from build123d import *

# Parameters (mm, degrees)
BOSS_EXTRUDE1_DEPTH = 4
SKETCH4_R           = 1.5
CUT_EXTRUDE1_DEPTH  = 3
SKETCH5_R           = 1.5
CUT_EXTRUDE2_DEPTH  = 3
SKETCH6_W           = 14.4
SKETCH6_H           = 0.4
CUT_EXTRUDE3_DEPTH  = 4
FILLET1_R           = 1
FILLET2_R           = 2


with BuildPart() as part:
    # Sketch3 → Boss-Extrude1 (new body)
    with BuildSketch(Plane(origin=(0, 0, 0), x_dir=(0, 1, 0), z_dir=(0, 0, 1))):
        with BuildLine():
            Line((-34.7, -0.521026003), (-34.7, -2.457826354))
            ThreePointArc((-34.7, -2.457826354), (-37.7, -4.907316097), (-34.7, -7.35680584))
            Line((-34.7, -7.35680584), (-34.7, -9.880280288))
            Line((-34.7, -9.880280288), (-34.7, -32.518065271))
            ThreePointArc((-34.7, -32.518065271), (-37.5, -35), (-34.7, -37.481934729))
            Line((-34.7, -37.481934729), (-34.7, -42.857826354))
            ThreePointArc((-34.7, -42.857826354), (-37.7, -45.307316097), (-34.7, -47.75680584))
            Line((-34.7, -47.75680584), (-34.7, -48.807316097))
            Line((-34.7, -48.807316097), (34.7, -48.807316097))
            Line((34.7, -48.807316097), (34.7, -47.75680584))
            ThreePointArc((34.7, -47.75680584), (37.7, -45.307316097), (34.7, -42.857826354))
            Line((34.7, -42.857826354), (34.7, -37.481934729))
            ThreePointArc((34.7, -37.481934729), (37.5, -35), (34.7, -32.518065271))
            Line((34.7, -32.518065271), (34.7, -7.35680584))
            ThreePointArc((34.7, -7.35680584), (37.7, -4.907316097), (34.7, -2.457826354))
            Line((34.7, -2.457826354), (34.7, -0.521026003))
            Line((34.7, -0.521026003), (6.445103659, -0.521026003))
            ThreePointArc((6.445103659, -0.521026003), (4, 2.5), (1.554896341, -0.521026003))
            Line((1.554896341, -0.521026003), (-1.554896341, -0.521026003))
            ThreePointArc((-1.554896341, -0.521026003), (-4, 2.5), (-6.445103659, -0.521026003))
            Line((-6.445103659, -0.521026003), (-34.7, -0.521026003))
        make_face()
        Polygon((-32.7, -9.880280288), (-32.7, -46.807316097), (32.7, -46.807316097), (32.7, -2.521026003), (-32.7, -2.521026003), align=None, mode=Mode.SUBTRACT)
    extrude(amount=BOSS_EXTRUDE1_DEPTH)

    # Sketch4 → Cut-Extrude1 (cut)
    with BuildSketch(Plane.XY.offset(4)):
        with Locations((0, 4)):
            Circle(SKETCH4_R)
        with Locations((0, -4)):
            Circle(SKETCH4_R)
        with Locations((35, -35)):
            Circle(SKETCH4_R)
        with Locations((35, 35)):
            Circle(SKETCH4_R)
    extrude(amount=-CUT_EXTRUDE1_DEPTH, mode=Mode.SUBTRACT)

    # Sketch5 → Cut-Extrude2 (cut)
    with BuildSketch(Plane(origin=(0, 0, 0), x_dir=(1, 0, 0), z_dir=(0, 0, -1))):
        with Locations(Location((4.907316097, 35.2, 0), (0, 0, 180))):
            Circle(SKETCH5_R)
        with Locations(Location((45.307316097, 35.2, 0), (0, 0, 180))):
            Circle(SKETCH5_R)
        with Locations(Location((45.307316097, -35.2, 0), (0, 0, 180))):
            Circle(SKETCH5_R)
        with Locations(Location((4.907316097, -35.2, 0), (0, 0, 180))):
            Circle(SKETCH5_R)
    extrude(amount=-CUT_EXTRUDE2_DEPTH, mode=Mode.SUBTRACT)

    # Sketch6 → Cut-Extrude3 (cut)
    with BuildSketch(Plane.XY.offset(4)):
        with Locations((9.721026003, -32.9)):
            Rectangle(SKETCH6_W, SKETCH6_H)
    extrude(amount=-CUT_EXTRUDE3_DEPTH, mode=Mode.SUBTRACT)

    # Fillet1
    fillet1_edges = [part.edges().sort_by_distance(p)[0] for p in [
        (2.457826354, -34.7, 2),
        (0.521026003, -6.445103659, 2),
        (0.521026003, -1.554896341, 2),
        (0.521026003, 1.554896341, 2),
        (0.521026003, 6.445103659, 2),
        (2.457826354, 34.7, 2),
        (7.35680584, 34.7, 2),
        (32.518065271, 34.7, 2),
        (37.481934729, 34.7, 2),
        (42.857826354, 34.7, 2),
        (47.75680584, 34.7, 2),
        (47.75680584, -34.7, 2),
        (42.857826354, -34.7, 2),
        (37.481934729, -34.7, 2),
        (32.518065271, -34.7, 2),
        (7.35680584, -34.7, 2),
    ]]
    fillet(fillet1_edges, radius=FILLET1_R)

    # Fillet2
    fillet2_edges = [part.edges().sort_by_distance(p)[0] for p in [
        (0.521026003, 34.7, 2),
        (48.807316097, 34.7, 2),
        (48.807316097, -34.7, 2),
        (0.521026003, -34.7, 2),
    ]]
    fillet(fillet2_edges, radius=FILLET2_R)


solid = part.part
Design review of the part built by this model. Coordinates are the model's own, in mm. A direction names the side the tool comes from. Round coordinates to 2 decimals unless told otherwise and drop trailing zeros. Write each loop counter-clockwise with the first axis right and the second up, starting at its lowest first coordinate (ties: lowest second). Pieces come first, ordered by that corner, then holes. Notation, with made-up numbers: (33.5, 16.25) - (79.5, 16.25) arc R9 cw to (79.5, 30.25) - close; hole circle Ø9 at (13.25, 37). An arc over 180 degrees is marked (long way). Use a Markdown table: item, result. Add a question column.
1. We need section B-B (x = 23). State the section outline as (y, z) points, then the cut area to 3 significant figures.
2. Clearance check with flat-ended pins moving along their axes: pin 1 (0.9 mm diameter, centred on y = 0, z = 1.5, fed in from -X); pin 2 (1.5 mm diameter, centred on x = 5, y = 35.5, fed in from -Z); pin 3 (1.5 mm diameter, centred on x = 0, y = -3.5, fed in from +Z). State where each tip first meets the part, or that it passes through.
3. For faces 1 (the face through (10, -33.1, 2)), 2 (the face through (0, 4, 1)), 3 (the face through (45, -35, 3)), 4 (the face through (0.521, -20, 2)), list the 3-axis set-ups (+Z, -Z, +X, -X, +Y, -Y) from which the entire face can be reached by the end or side of a thin tool; tool diameter is ignored.
4. We need section A-A (y = 4). State the section outline as (x, z) points, then the cut area to 3 significant figures.
5. We need section C-C (y = -14). State the section outline as (x, z) points.
6. We need section D-D (x = 35). State the section outline as (y, z) points.
7. Wall thickness on probe 1 along Y at (x, z) = (35, 2.95); probe 2 along Y at (x, z) = (5, 3.6); probe 3 along X at (y, z) = (-25, 1.05): over which ranges is each line inside the solid? List them lowest first.
8. Mouldability with a two-part tool opening along X and no side actions: class faces 5 (the face through (45, 35, 3)), 6 (the face through (2, 0, 4)), 7 (the face through (-2.5, 4.1, 2)) as +X half, -X half, draft (parallel to the pull), parting line (faces both ways), or undercut.
Output:
| question | item | result |
|---|---|---|
| 1 | outline | (-34.7, 0) - (-32.7, 0) - (-32.7, 4) - (-34.7, 4) - close; (32.7, 0) - (34.7, 0) - (34.7, 4) - (32.7, 4) - close |
| 1 | area | 16.0 mm2 |
| 2 | pin 1 | stops at x = 0.52 |
| 2 | pin 2 | stops at z = 3 |
| 2 | pin 3 | stops at z = 1 |
| 3 | face 1 | +Z, -Z |
| 3 | face 2 | +Z |
| 3 | face 3 | -Z |
| 3 | face 4 | +Z, -Z, -X, -Y |
| 4 | outline | (-2.5, 0) - (2.52, 0) - (2.52, 4) - (1.5, 4) - (1.5, 1) - (-1.5, 1) - (-1.5, 4) - (-2.5, 4) - close; (46.81, 0) - (48.81, 0) - (48.81, 4) - (46.81, 4) - close |
| 4 | area | 19.1 mm2 |
| 5 | outline | (0.52, 0) - (2.52, 0) - (2.52, 4) - (0.52, 4) - close; (46.81, 0) - (48.81, 0) - (48.81, 4) - (46.81, 4) - close |
| 6 | outline | (-37.5, 0) - (-32.7, 0) - (-32.7, 4) - (-33.5, 4) - (-33.5, 1) - (-36.5, 1) - (-36.5, 4) - (-37.5, 4) - close; (32.7, 0) - (37.5, 0) - (37.5, 4) - (36.5, 4) - (36.5, 1) - (33.5, 1) - (33.5, 4) - (32.7, 4) - close |
| 7 | probe 1 | y = -37.5 to -36.5, -33.5 to -32.7, 32.7 to 33.5, 36.5 to 37.5 |
| 7 | probe 2 | y = -37.7 to -33.1, 32.7 to 37.7 |
| 7 | probe 3 | x = 0.52 to 2.52, 46.81 to 48.81 |
| 8 | face 5 | undercut |
| 8 | face 6 | draft |
| 8 | face 7 | -X half |
